```python
from build123d import *

# Parameters (mm, degrees)
SKETCH297_R       = 1
PAD079_DEPTH      = 6
PAD079_DEPTH_BACK = 4
SKETCH298_R       = 2.35
SKETCH298_R_2     = 1.1
PAD082_DEPTH      = 6
CHAMFER003_SIZE   = 0.4


with BuildPart() as part:
    # Sketch297 → Pad079 (new body, two sides)
    with BuildSketch(Plane.XY) as pad079_sk:
        with BuildLine():
            ThreePointArc((-100.991564, 102.241564), (-101.875447, 101.875447), (-102.241564, 100.991564))
            Line((-102.241564, 61.991564), (-102.241564, 100.991564))
            ThreePointArc((-102.241564, 61.991564), (-101.875447, 61.107681), (-100.991564, 60.741564))
            Line((-61.991564, 60.741564), (-100.991564, 60.741564))
            ThreePointArc((-61.991564, 60.741564), (-61.107681, 61.107681), (-60.741564, 61.991564))
            Line((-60.741564, 100.991564), (-60.741564, 61.991564))
            ThreePointArc((-60.741564, 100.991564), (-61.107681, 101.875447), (-61.991564, 102.241564))
            Line((-100.991564, 102.241564), (-61.991564, 102.241564))
        make_face()
        with Locations((-73.539105, 73.539105)):
            Circle(SKETCH297_R, mode=Mode.SUBTRACT)
    extrude(amount=PAD079_DEPTH)
    extrude(pad079_sk.sketch, amount=-PAD079_DEPTH_BACK)

    # Sketch301 → Groove008 (revolve, cut)
    with BuildSketch(Plane.XZ):
        with BuildLine():
            Line((-96.7, 7), (0, 7))
            Line((0, 0), (0, 7))
            Line((-93.7, 0), (0, 0))
            ThreePointArc((-96.7, 3), (-95.82132, 0.87868), (-93.7, 0))
            Line((-96.7, 7), (-96.7, 3))
        make_face()
        Polygon((-165, 7), (-98.5, 7), (-98.5, 0), (-110, 0), (-111.4, -1.4), (-144.1, -1.4), (-145.5, 0), (-165, 0), align=None)
    revolve(axis=Axis((0, 0, 0), (0, 0, 1)), mode=Mode.SUBTRACT)

    # Sketch298 → Pad082 (join)
    with BuildSketch(Plane.XY):
        with Locations((-73.539105, 73.539105)):
            Circle(SKETCH298_R)
        with Locations((-73.539105, 73.539105)):
            Circle(SKETCH298_R_2, mode=Mode.SUBTRACT)
    extrude(amount=PAD082_DEPTH)

    # Chamfer003
    chamfer003_edges = [part.edges().sort_by_distance(p)[0] for p in [
        (-101.875447, 101.875447, -4),
        (-102.241564, 81.491564, -4),
        (-101.875447, 61.107681, -4),
        (-81.491564, 60.741564, -4),
        (-61.107681, 61.107681, -4),
        (-60.741564, 81.491564, -4),
        (-61.107681, 101.875447, -4),
        (-81.491564, 102.241564, -4),
        (-74.539105, 73.539105, -4),
        (-77.541682, 60.741564, 3),
        (-60.741564, 77.541682, 3),
    ]]
    chamfer(chamfer003_edges, length=CHAMFER003_SIZE)


with BuildPart() as part_1:
    # Body022063 placement: moved
    add(part.part.moved(Location((0, 0, -153))))


solid = part_1.part
```
Work out the finished part from the listing and answer in its coordinate system (mm). A direction names the side the tool comes from. Give positions to 0.01 mm unless a question says otherwise; leave off trailing zeros. Loops run counter-clockwise (first coordinate to the right, second up) from the corner with the lowest first, then second, coordinate; pieces in that order, holes last. Notation, with made-up numbers: (24.5, 81.5) - (55.5, 81.5) arc R12 ccw to (55.5, 89.5) - close; hole circle Ø1 at (-29, -23.5). An arc over 180 degrees is marked (long way). Use CSV: the item, a comma, the result in double quotes. Start each with the question number.
(1) Each of these flat-tipped pins is pushed along its axis until it touches: pin 1 (5.5 mm diameter, centred on x = -68, y = 65.5, fed in from +Z); pin 2 (4 mm diameter, centred on x = -72.5, y = 88.5, fed in from +Z); pin 3 (5 mm diameter, centred on x = -78.5, y = 81, fed in from +Z). Where does it stop, or does it pass through?
(2) Find section B-B, the plane y = 100.5. Determine the outline of the cut face in (x, z), plus the area to 3 significant figures.
(3) Determine the mould class of faces 1 (the face through (-69.5, 69.8, -150)), 2 (the face through (-101.708, 61.29, -156.847)), 3 (the face through (-75, 73, -147)) for opening direction Y: released by +Y, released by -Y, zero draft, split by the parting line, or undercut.
(4) A tool of negligible diameter and unlimited length cuts with its end or side. For faces 4 (the face through (-61.29, 61.275, -156.847)), 5 (the face through (-86, 86, -154.4)), 6 (the face through (-68.275, 68.479, -148.521)), 7 (the face through (-81, 60.742, -154)), 8 (the face through (-72.5, 73.9, -150)), from which of +Z, -Z, +X, -X, +Y, -Y can it reach the whole face along a straight path? Write none if from no direction.
(5) Find section C-C, the plane z = -153.5. Determine the outline of the cut face in (x, y), plus the area to 3 significant figures.
(6) Find section A-A, the plane x = -94.5. Determine the outline of the cut face in (y, z), plus the area to 3 significant figures.
(7) Find the intervals of material crossed by L1, parallel to Z at x = -75, y = 71.5; L2, parallel to Z at x = -84.5, y = 86.5; L3, parallel to Y at x = -73, z = -149.5, in increasing order.
Results found:
1,pin 1,"z = -147"
1,pin 2,"z = -154.4"
1,pin 3,"z = -153.3"
2,outline,"(-102.24, -156.6) - (-101.84, -157) - (-61.14, -157) - (-60.74, -156.6) - (-60.74, -154.4) - (-102.24, -154.4) - close"
2,area,"108 mm^2"
3,face 1,"undercut"
3,face 2,"released by -Y"
3,face 3,"zero draft"
4,face 4,"-Z, +X, -Y"
4,face 5,"+Z, -X, +Y"
4,face 6,"+Z, +X, -Y"
4,face 7,"+Z, -Z, +X, -X, -Y"
4,face 8,"+Z"
5,outline,"(-92.31, 60.74) - (-61.99, 60.74) arc R1.25 ccw to (-60.74, 61.99) - (-60.74, 92.31) arc R110.5 ccw to start; hole circle Ø2 at (-73.54, 73.54)"
5,area,"563 mm^2"
6,outline,"(60.74, -156.6) - (61.14, -157) - (101.84, -157) - (102.24, -156.6) - (102.24, -154.4) - (60.74, -154.4) - close"
6,area,"108 mm^2"
7,L1,"-157 to -153"
7,L2,"-157 to -154.4"
7,L3,"63.42 to 66.13, 71.25 to 72.58, 74.5 to 75.83"
